from build123d import *

# Parameters (mm, degrees)
SKETCH1_W           = 228
SKETCH1_H           = 165
BOSS_EXTRUDE1_DEPTH = 70
SKETCH2_OUTSIDE_W   = 288.004
SKETCH2_OUTSIDE_H   = 225.004
SKETCH2_OUTSIDE_W_2 = 228
SKETCH2_OUTSIDE_H_2 = 165
SKETCH2_OUTSIDE_W_3 = 224
SKETCH2_OUTSIDE_H_3 = 161
CUT_EXTRUDE1_DEPTH  = 68


with BuildPart() as part:
    # Sketch1 → Boss-Extrude1 (new body)
    with BuildSketch(Plane(origin=(0, 0, 0), x_dir=(1, 0, 0), z_dir=(0, 1, 0))):
        with Locations((17.256257449, -4.235399285)):
            Rectangle(SKETCH1_W, SKETCH1_H)
    extrude(amount=BOSS_EXTRUDE1_DEPTH)

    # Sketch2 outside → Cut-Extrude1 (cut)
    # profile 1 of 2: a face of its own
    with BuildSketch(Plane(origin=(0, 70, 0), x_dir=(1, 0, 0), z_dir=(0, 1, 0))):
        with Locations((17.256, -4.235)):
            Rectangle(SKETCH2_OUTSIDE_W, SKETCH2_OUTSIDE_H)
        with Locations((17.256257449, -4.235399285)):
            Rectangle(SKETCH2_OUTSIDE_W_2, SKETCH2_OUTSIDE_H_2, mode=Mode.SUBTRACT)
    # profile 2 of 2: a face of its own
    with BuildSketch(Plane(origin=(0, 70, 0), x_dir=(1, 0, 0), z_dir=(0, 1, 0))):
        with Locations((17.256257449, -4.235399285)):
            Rectangle(SKETCH2_OUTSIDE_W_3, SKETCH2_OUTSIDE_H_3)
    extrude(amount=-CUT_EXTRUDE1_DEPTH, mode=Mode.SUBTRACT)


solid = part.part
Part model, mm, in its own coordinate system. A direction names the side the tool comes from. Give positions to 0.01 mm unless a question says otherwise; leave off trailing zeros. Order: outer loops, then holes, each group sorted by start corner. A loop starts at its lowest first (then second) coordinate and runs counter-clockwise, first axis right, second up. Notation, with made-up numbers: (-23, 67) - (17, 67) arc R7 cw to (17, 80) - close; hole circle Ø2 at (74.5, -22). An arc over 180 degrees is marked (long way). Use a Markdown table: item, result.
1) Saw through at A-A on y = 62.5. List the corners of the cut face in (x, z), plus the area to 3 significant figures.
Checked values:
| item | result |
|---|---|
| outline | (-96.74, -78.26) - (131.26, -78.26) - (131.26, 86.74) - (-96.74, 86.74) - close; hole (-94.74, -76.26) - (129.26, -76.26) - (129.26, 84.74) - (-94.74, 84.74) - close |
| area | 1,560 mm² |
2) Saw through at B-B on z = 19.5. List the corners of the cut face in (x, y), plus the area to 3 significant figures.
Checked values:
| item | result |
|---|---|
| outline | (-96.74, 0) - (131.26, 0) - (131.26, 70) - (129.26, 70) - (129.26, 2) - (-94.74, 2) - (-94.74, 70) - (-96.74, 70) - close |
| area | 728 mm² |
3) Flat gauge pins, fed straight in: P1, Ø8, axis at x = 24.5, z = 32.5, coming from the +Y side; P2, Ø5, axis at x = -43.5, z = 58, coming from the -Y side. Where does each tip first touch, or does it go through?
Checked values:
| item | result |
|---|---|
| P1 | y = 2 |
| P2 | y = 0 |
4) 3-axis set-ups, long thin cutter, end or side, ignore diameter. For faces 1 (the flat face through (129.256, 36, 5)), 2 (the flat face through (16, 35, 86.735)): which of +Z, -Z, +X, -X, +Y, -Y reach the whole face in a straight line?
Checked values:
| item | result |
|---|---|
| face 1 | +Y |
| face 2 | +Z, +X, -X, +Y, -Y |
5) Saw through at C-C on x = -5. List the corners of the cut face in (y, z).
Checked values:
| item | result |
|---|---|
| outline | (0, -78.26) - (70, -78.26) - (70, -76.26) - (2, -76.26) - (2, 84.74) - (70, 84.74) - (70, 86.74) - (0, 86.74) - close |
6) Probe L1, parallel to Z at x = 101, y = 64; L2, parallel to X at y = 53, z = -7.5; L3, parallel to Y at x = -18.5, z = 41. List the from-to ranges inside material, lowest first. Write a range as from..to.
Checked values:
| item | result |
|---|---|
| L1 | -78.26..-76.26, 84.74..86.74 |
| L2 | -96.74..-94.74, 129.26..131.26 |
| L3 | 0..2 |
